Can you work these out from the model? Positions are in its coordinate system, mm. Face numbers are marked on the shaded views. A direction names the side the tool comes from. Give positions to 0.01 mm unless a question says otherwise; leave off trailing zeros. Write each loop counter-clockwise with the first axis right and the second up, starting at its lowest first coordinate (ties: lowest second). Pieces come first, ordered by that corner, then holes.
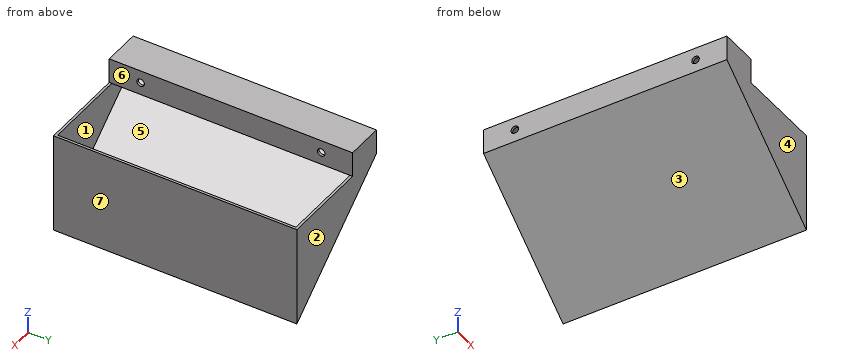
Autodesk Inventor part; units mm, degrees
ref_plane "YZ Plane" through (0, 0, 0) normal (1, 0, 0) x (0, 1, 0)
ref_plane "XZ Plane" through (0, 0, 0) normal (0, 1, 0) x (-1, 0, 0)
ref_plane "XY Plane" through (0, 0, 0) normal (0, 0, 1) x (1, 0, 0)
sketch "Esboço1" plane through (0, 0, 0) normal (0, 1, 0) x (-1, 0, 0)
  line L0 (0, 20) -> (0, -20)
  line L1 (0, 20) -> (50, 20)
  line L2 (50, 20) -> (0, -20)
  line L3 (50, 20) -> (50, 30)
  line L4 (50, 30) -> (35, 30)
  line L5 (35, 30) -> (35, 20)
  point P0 (0, 0)
  dimension "d0" = 40
  dimension "d1" = 50
  dimension "d2" = 10
  dimension "d3" = 15
extrude "Extrusão1" add sketch "Esboço1" along normal blind 97.084
shell "Casca1" thickness 1 removed faces 1 at (-23.3333, 32.3613, 20)
sketch "Esboço2" plane through (-50, 0, 20) normal (-1, 0, 0) x (0, 0, 1)
  line L0 (10, 97.084) -> (0, 97.084)
  line L1 (0, 97.084) -> (5, 97.084)
  line L2 (5, 97.084) -> (5, 84.584)
  circle A0 centre (5, 84.584) radius 1.5
  line L3 (10, 0) -> (0, 0)
  line L4 (0, 0) -> (5, 0)
  line L5 (5, 0) -> (5, 12.5)
  circle A1 centre (5, 12.5) radius 1.5
  point P0 (-20, 0)
  dimension "d7" = 5
  dimension "d8" = 12.5
  dimension "d9" = 3
  dimension "d10" = 5
  dimension "d11" = 12.5
  dimension "d12" = 3
extrude "Extrusão2" cut sketch "Esboço2" against normal blind 102.84
thread "Rosca1"
thread "Rosca2"
thread "Rosca3"
thread "Rosca4"
sketch "Esboço3" plane through (0, 97.084, 0) normal (0, 1, 0) x (1, 0, 0)
  line L0 (-50, -30) -> (-35, -30)
  point P0 (0, 0)
  point P1 (-35, -20)
  dimension "d23" = 10
sketch "Esboço4" plane through (-50, 0, 20) normal (-1, 0, 0) x (0, 0, 1)
  line L0 (0, 97.084) -> (10, 97.084)
  line L1 (0, 0) -> (10, 0)
  point P0 (-20, 0)
  dimension "d24" = 97.084
sketch "Esboço5" plane through (0, 97.084, 0) normal (0, 1, 0) x (1, 0, 0)
  point P0 (0, 0)
properties part number "Rampa 1"
1) For the marked faces 5, 6 and 7, which set-ups out of +Z, -Z, +X, -X, +Y, -Y let a thin tool reach every point of the face, with its end or its side?
Values follow:
face 5: none
face 6: +Z, +X, +Y, -Y
face 7: +Z, -Z, +X, +Y, -Y
2) If we mould it in two halves opening along Y, with no side actions, what happens to the marked faces 1, 2, 3 and 4? For each: +Y half, -Y half, draft (parallel to the pull), parting line (faces both ways), or undercut.
Values follow:
face 1: undercut
face 2: +Y half
face 3: draft
face 4: -Y half
3) Suppose I cut it at B-B on z = 25. Write out the boundary of the cut face in (x, y), plus the area to 3 significant figures.
Values follow:
outline: (-50, 0) - (-35, 0) - (-35, 11) - (-36, 11) - (-36, 1) - (-49, 1) - (-49, 11) - (-50, 11) - close; (-50, 14) - (-49, 14) - (-49, 83.08) - (-50, 83.08) - close; (-50, 86.08) - (-49, 86.08) - (-49, 96.08) - (-36, 96.08) - (-36, 86.08) - (-35, 86.08) - (-35, 97.08) - (-50, 97.08) - close; (-36, 14) - (-35, 14) - (-35, 83.08) - (-36, 83.08) - close
area: 208 mm2
4) Please list where these lines run through material, in increasing order: L1, parallel to Y at x = -35.3, z = 25; L2, parallel to Y at x = -4.5, z = -11; L3, parallel to Z at x = -40.5, y = 29.5.
Values follow:
L1: y = 0 to 11, 14 to 83.08, 86.08 to 97.08
L2: y = 0 to 1, 96.08 to 97.08
L3: z = 12.4 to 13.68, 29 to 30
5) For pin 1 Ø11.5 at (y, z) = (61.5, -2) entering from -X; pin 2 Ø1 at (x, y) = (-31, 23.5) entering from +Z; pin 3 Ø1.5 at (y, z) = (86.5, 16.5) entering from -X, each with a flat end and sliding along its axis, tell me the tip position at first contact or that it passes through.
Values follow:
pin 1: stops at x = -29.69
pin 2: stops at z = 6.48
pin 3: stops at x = -46.56
6) Suppose I cut it at C-C on z = -4. Write out the boundary of the cut face in (x, y).
Values follow:
outline: (-20, 0) - (0, 0) - (0, 97.08) - (-20, 97.08) - close; hole (-18.4, 1) - (-1, 1) - (-1, 96.08) - (-18.4, 96.08) - close
7) Suppose I cut it at A-A on y = 12.5. Write out the boundary of the cut face in (x, z).
Values follow:
outline: (-50, 20) - (0, -20) - (0, 20) - (-1, 20) - (-1, -17.92) - (-49, 20.48) - (-49, 23.5) - (-50, 23.5) - close; (-50, 26.5) - (-49, 26.5) - (-49, 29) - (-36, 29) - (-36, 26.5) - (-35, 26.5) - (-35, 30) - (-50, 30) - close; (-36, 20) - (-35, 20) - (-35, 23.5) - (-36, 23.5) - close
8) Suppose I cut it at D-D on x = -8. Write out the boundary of the cut face in (y, z).
Values follow:
outline: (0, -13.6) - (97.08, -13.6) - (97.08, 20) - (96.08, 20) - (96.08, -12.32) - (1, -12.32) - (1, 20) - (0, 20) - close
